Check sheet for the modelled part. Datum: model origin and axes. Units: mm. Face numbers are marked on the shaded views. Round coordinates to 2 decimals unless told otherwise and drop trailing zeros. Write each loop counter-clockwise with the first axis right and the second up, starting at its lowest first coordinate (ties: lowest second). Pieces come first, ordered by that corner, then holes. Notation, with made-up numbers: M 42.25,-28.75 L 57.25,-28.75 A10 cw 57.25,-24.75 Z; hole C -32,-36.75 d6. An arc over 180 degrees is marked long. One line per item, written item: value.
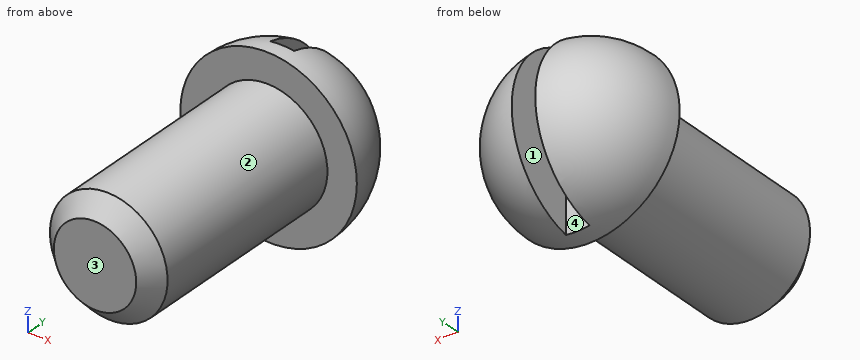
from build123d import *

# Parameters (mm, degrees)
SKETCH6_W          = 4
SKETCH6_H          = 15
CUT_EXTRUDE1_DEPTH = 27.5
CHAMFER1_SIZE      = 3


with BuildPart() as part:
    # Sketch4 → Revolve1 (revolve)
    with BuildSketch(Plane.XY):
        with BuildLine():
            Line((0, 0), (10, 0))
            Line((10, 0), (10, 53))
            ThreePointArc((10, 53), (-0.606601718, 48.606601718), (-5, 38))
            Line((-5, 38), (0, 38))
            Line((0, 38), (0, 0))
        make_face()
    revolve(axis=Axis((10, -13.659497016, 0), (0, 1, 0)))

    # Sketch6 → Cut-Extrude1 (cut, symmetric)
    with BuildSketch(Plane.XY):
        with Locations((10, 48.5)):
            Rectangle(SKETCH6_W, SKETCH6_H)
    extrude(amount=CUT_EXTRUDE1_DEPTH, both=True, mode=Mode.SUBTRACT)

    # Chamfer1
    chamfer1_edges = [part.edges().sort_by_distance(p)[0] for p in [
        (20, 0, 0),
    ]]
    chamfer(chamfer1_edges, length=CHAMFER1_SIZE)


solid = part.part
Q1. Sectioned sample at A-A on z = 0. Enter the section's corners in (x, y).
Completed:
outline: M -5,38 L 0,38 L 0,3 L 3,0 L 17,0 L 20,3 L 20,38 L 25,38 A15 ccw 12,52.87 L 12,41 L 8,41 L 8,52.87 A15 ccw Z
Q2. Sectioned sample at C-C on y = 44. Enter the section's corners in (x, z).
Completed:
outline: M 8,-13.6 L 8,13.6 A13.75 ccw Z; M 12,-13.6 A13.75 ccw 12,13.6 Z
Q3. Draft check along X on the marked faces 1, 2, 3 and 4. Enter one of: pulls with the +X half, pulls with the -X half, needs draft (parallel to the pull), parting line crosses it, or undercut.
Completed:
face 1: undercut
face 2: parting line crosses it
face 3: needs draft
face 4: undercut
Q4. Scan lines: line 1 (X direction, y = 29.5, z = 0.5); line 2 (Y direction, x = 8.75, z = -12.5); line 3 (Z direction, x = 17, y = 7.5). Record each from-to range of solid material in increasing order. Write a range as [from, to].
Completed:
line 1: [0.01, 19.99]
line 2: [38, 41]
line 3: [-7.14, 7.14]
Q5. Depth check by flat-ended pin: P1, Ø12, axis at y = 11, z = 11.5, coming from the +X side; P2, Ø5, axis at x = 16, y = 17.5, coming from the -Z side; P3, Ø6, axis at x = -1, y = 24, coming from the +Z side. Enter the tip coordinate at first touch or a pass-through.
Completed:
P1: x = 18.35
P2: z = -9.37
P3: z = 6
Q6. Sectioned sample at D-D on y = 11. Enter the section's corners in (x, z), and give its area (3 significant figures).
Completed:
outline: C 10,0 d20
area: 314 mm^2
Q7. Sectioned sample at B-B on x = 10. Enter the section's corners in (y, z).
Completed:
outline: M 0,-7 L 3,-10 L 38,-10 L 38,-15 A15 ccw 41,-14.7 L 41,14.7 A15 ccw 38,15 L 38,10 L 3,10 L 0,7 Z
